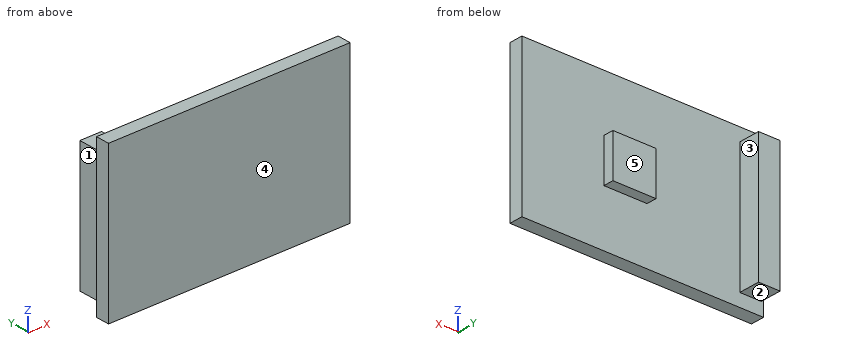
```python
from build123d import *

# Parameters (mm, degrees)
SKETCH1_W          = 28
SKETCH1_H          = 18
PCB_DEPTH          = 1.6
ADS1115_CHIP_START = 1.6
SKETCH2_W          = 5
SKETCH2_H          = 5
ADS1115_CHIP_DEPTH = 1.2
HEADER_START       = 1.6
SKETCH3_W          = 2.5
SKETCH3_H          = 15
HEADER_DEPTH       = 2.5


with BuildPart() as part:
    # Sketch1 → PCB (new body)
    with BuildSketch(Plane(origin=(0, 0, 0), x_dir=(1, 0, 0), z_dir=(0, 1, 0))):
        Rectangle(SKETCH1_W, SKETCH1_H)
    extrude(amount=PCB_DEPTH)

    # Sketch2 → ADS1115_Chip (add)
    with BuildSketch(Plane(origin=(0, 0, 0), x_dir=(1, 0, 0), z_dir=(0, 1, 0)).offset(ADS1115_CHIP_START)):
        with Locations((2, 0)):
            Rectangle(SKETCH2_W, SKETCH2_H)
    extrude(amount=ADS1115_CHIP_DEPTH)

    # Sketch3 → Header (add)
    with BuildSketch(Plane(origin=(0, 0, 0), x_dir=(1, 0, 0), z_dir=(0, 1, 0)).offset(HEADER_START)):
        with Locations((-12.5, 0)):
            Rectangle(SKETCH3_W, SKETCH3_H)
    extrude(amount=HEADER_DEPTH)


solid = part.part
```
Geometry: final body of the model. Coordinates: model frame, mm. Face numbers are marked on the shaded views. A direction names the side the tool comes from. Coordinates: 2 decimals unless noted, no trailing zeros. Order: outer loops, then holes, each group sorted by start corner. A loop starts at its lowest first (then second) coordinate and runs counter-clockwise, first axis right, second up. Notation, with made-up numbers: M 41.5,42.5 L 56.5,42.5 A4 cw 56.5,48.5 Z; hole C 42,-35.75 d7. An arc over 180 degrees is marked long. Answer as CSV lines item,"result".
Q1. Draft query along X for the marked faces 1, 2 and 3. Return one class per face: pulls with the +X half, pulls with the -X half, needs draft (parallel to the pull), parting line crosses it, or undercut.
Answers:
face 1,"pulls with the -X half"
face 2,"needs draft"
face 3,"undercut"
Q2. First-contact query: P1, Ø1.5, axis at x = -3.5, z = 6.5, coming from the +Y side; P2, Ø2.5, axis at x = 1, z = -1, coming from the +Y side; P3, Ø1.3, axis at x = 1, y = 2.5, coming from the -Z side. Flat tips, straight axial feed; report the tip coordinate or a pass-through.
Answers:
P1,"stops at y = 1.6"
P2,"stops at y = 2.8"
P3,"stops at z = -2.5"
Q3. Section D-D on z = -1.5. Return the cut outline in (x, y).
Answers:
outline,"M -14,0 L 14,0 L 14,1.6 L 4.5,1.6 L 4.5,2.8 L -0.5,2.8 L -0.5,1.6 L -11.25,1.6 L -11.25,4.1 L -13.75,4.1 L -13.75,1.6 L -14,1.6 Z"
Q4. Section B-B on x = 0.5. Return the cut outline in (y, z).
Answers:
outline,"M 0,-9 L 1.6,-9 L 1.6,-2.5 L 2.8,-2.5 L 2.8,2.5 L 1.6,2.5 L 1.6,9 L 0,9 Z"
Q5. Section A-A on y = 2.25. Return the cut outline in (x, z).
Answers:
outline,"M -13.75,-7.5 L -11.25,-7.5 L -11.25,7.5 L -13.75,7.5 Z; M -0.5,-2.5 L 4.5,-2.5 L 4.5,2.5 L -0.5,2.5 Z"
Q6. Section C-C on z = -4.25. Return the cut outline in (x, y).
Answers:
outline,"M -14,0 L 14,0 L 14,1.6 L -11.25,1.6 L -11.25,4.1 L -13.75,4.1 L -13.75,1.6 L -14,1.6 Z"
Q7. Line query: probe 1 along X at (y, z) = (1.85, 1.5); probe 2 along X at (y, z) = (2.3, 5.5); probe 3 along Y at (x, z) = (-8.75, -8). Output: solid intervals per line, ascending. Write a range as [from, to].
Answers:
probe 1,"x = [-13.75, -11.25], [-0.5, 4.5]"
probe 2,"x = [-13.75, -11.25]"
probe 3,"y = [0, 1.6]"
Q8. Set-up query: the marked faces 4 and 5. Return all of +Z, -Z, +X, -X, +Y, -Y with unobstructed straight access to the full face (end or side cutting, diameter ignored); none if empty.
Answers:
face 4,"+Z, -Z, +X, -X, -Y"
face 5,"+Z, -Z, +X, +Y"
